```python
from build123d import *

# Parameters (mm, degrees)
SKETCH_1_R               = 2.5
EXTRUDE_1_DEPTH          = 4
SKETCH_3_R               = 7.5
EXTRUDE_3_DEPTH          = 6
SKETCH_4_R               = 10
EXTRUDE_4_DEPTH          = 5
SKETCH_5_R               = 3.175
EXTRUDE_5_DEPTH          = 11
SKETCH_6_R               = 10
EXTRUDE_6_DEPTH          = 5
SKETCH_7_R               = 7.5
EXTRUDE_7_DEPTH          = 7
SKETCH_8_R               = 2.5
EXTRUDE_8_DEPTH          = 4
CUT_EXTRUDE_1_DEPTH      = 45.317039612
CUT_EXTRUDE_1_DEPTH_BACK = 1
SKETCH_10_R              = 2.5
SKETCH_13_R              = 10
SKETCH_13_R_2            = 2.5
CUT_EXTRUDE_3_DEPTH      = 15


with BuildPart() as part:
    # 草图1 → 凸台-拉伸1 (new body)
    with BuildSketch(Plane(origin=(0, 0, 0), x_dir=(1, 0, 0), z_dir=(0, 1, 0))):
        with Locations(Location((0, 0, 0), (0, 0, 270))):
            Circle(SKETCH_1_R)
    extrude(amount=EXTRUDE_1_DEPTH)

    # 草图3 → 凸台-拉伸3 (add)
    with BuildSketch(Plane(origin=(0, 4, 0), x_dir=(1, 0, 0), z_dir=(0, 1, 0))):
        with Locations(Location((0, 0, 0), (0, 0, 270))):
            Circle(SKETCH_3_R)
    extrude(amount=EXTRUDE_3_DEPTH)

    # 草图4 → 凸台-拉伸4 (add)
    with BuildSketch(Plane(origin=(0, 10, 0), x_dir=(1, 0, 0), z_dir=(0, 1, 0))):
        with Locations(Location((0, 0, 0), (0, 0, 270))):
            Circle(SKETCH_4_R)
    extrude(amount=EXTRUDE_4_DEPTH)

    # 草图5 → 凸台-拉伸5 (add)
    with BuildSketch(Plane(origin=(0, 15, 0), x_dir=(1, 0, 0), z_dir=(0, 1, 0))):
        with Locations(Location((0, 0, 0), (0, 0, 270))):
            Circle(SKETCH_5_R)
    extrude(amount=EXTRUDE_5_DEPTH)

    # 草图6 → 凸台-拉伸6 (add)
    with BuildSketch(Plane(origin=(0, 26, 0), x_dir=(1, 0, 0), z_dir=(0, 1, 0))):
        with Locations(Location((0, 0, 0), (0, 0, 270))):
            Circle(SKETCH_6_R)
    extrude(amount=EXTRUDE_6_DEPTH)

    # 草图7 → 凸台-拉伸7 (add)
    with BuildSketch(Plane(origin=(0, 31, 0), x_dir=(1, 0, 0), z_dir=(0, 1, 0))):
        with Locations(Location((0, 0, 0), (0, 0, 270))):
            Circle(SKETCH_7_R)
    extrude(amount=EXTRUDE_7_DEPTH)

    # 草图8 → 凸台-拉伸8 (add)
    with BuildSketch(Plane(origin=(0, 38, 0), x_dir=(1, 0, 0), z_dir=(0, 1, 0))):
        with Locations(Location((0, 0, 0), (0, 0, 270))):
            Circle(SKETCH_8_R)
    extrude(amount=EXTRUDE_8_DEPTH)

    # 草图10 → 切除-拉伸1 (cut, two sides: drawn at the far end of the back side and taken through both)
    with BuildSketch(Plane(origin=(0, 0, 0), x_dir=(-1, 0, 0), z_dir=(0, -1, 0)).offset(-CUT_EXTRUDE_1_DEPTH_BACK)):
        with Locations(Location((0, 0, 0), (0, 0, 90))):
            Circle(SKETCH_10_R)
    extrude(amount=CUT_EXTRUDE_1_DEPTH + CUT_EXTRUDE_1_DEPTH_BACK, mode=Mode.SUBTRACT)

    # 草图13 → 切除-拉伸3 (cut)
    with BuildSketch(Plane.XZ.offset(-26)):
        with Locations(Location((0, 0, 0), (0, 0, 90))):
            Circle(SKETCH_13_R)
        with Locations(Location((0, 0, 0), (0, 0, 270))):
            Circle(SKETCH_13_R_2, mode=Mode.SUBTRACT)
    extrude(amount=-CUT_EXTRUDE_3_DEPTH, mode=Mode.SUBTRACT)


solid = part.part
```
Input: part model. Units: mm. Frame: model coordinates. A direction names the side the tool comes from. Round coordinates to 2 decimals unless told otherwise and drop trailing zeros. Loops run counter-clockwise (first coordinate to the right, second up) from the corner with the lowest first, then second, coordinate; pieces in that order, holes last.
1) Pull-direction query (X, two-part tool) for faces 4 (the cylindrical face through (-1.93, 20.42, -2.52)), 5 (the flat face through (3, 26, 0)); classes: released by +X, released by -X, zero draft, split by the parting line, or undercut.
Ans:
face 4: split by the parting line
face 5: zero draft
2) Section query A-A on z = 0. Return the cut outline in (x, y) (3 decimals).
Ans:
outline: (-10, 10) - (-7.5, 10) - (-7.5, 4) - (-2.5, 4) - (-2.5, 1) - (2.5, 1) - (2.5, 4) - (7.5, 4) - (7.5, 10) - (10, 10) - (10, 15) - (3.175, 15) - (3.175, 26) - (2.5, 26) - (2.5, 42) - (-2.5, 42) - (-2.5, 26) - (-3.175, 26) - (-3.175, 15) - (-10, 15) - close
3) Section query C-C on y = 5. Return the cut outline in (x, z), plus the area to 3 significant figures.
Ans:
outline: circle Ø15 at (0, 0)
area: 177 mm2
4) Set-up query: faces 1 (the cylindrical face through (-2.44, 2.48, -0.54)), 2 (the flat face through (2.4, 15, -2.4)), 3 (the cylindrical face through (-9.76, 12.46, -2.17)). Return all of +Z, -Z, +X, -X, +Y, -Y with unobstructed straight access to the full face (end or side cutting, diameter ignored); none if empty.
Ans:
face 1: -Y
face 2: +Y
face 3: +Y, -Y
5) Pin query (flat end, axial travel): pin 1 (3 mm diameter, centred on y = 6.5, z = -3.5, fed in from -X); pin 2 (4 mm diameter, centred on x = 5.5, y = 6, fed in from +Z); pin 3 (5 mm diameter, centred on x = -4.5, y = 12, fed in from -Z). Return the tip coordinate at first contact, or that it passes through.
Ans:
pin 1: stops at x = -7.23
pin 2: stops at z = 6.63
pin 3: stops at z = -9.8
6) Section query D-D on z = 5.5. Return the cut outline in (x, y).
Ans:
outline: (-8.35, 10) - (-5.1, 10) - (-5.1, 4) - (5.1, 4) - (5.1, 10) - (8.35, 10) - (8.35, 15) - (-8.35, 15) - close
7) Section query B-B on x = -0.75. Return the cut outline in (y, z).
Ans:
outline: (1, -2.38) - (4, -2.38) - (4, -7.46) - (10, -7.46) - (10, -9.97) - (15, -9.97) - (15, -3.09) - (26, -3.09) - (26, -2.38) - (42, -2.38) - (42, 2.38) - (26, 2.38) - (26, 3.09) - (15, 3.09) - (15, 9.97) - (10, 9.97) - (10, 7.46) - (4, 7.46) - (4, 2.38) - (1, 2.38) - close
8) Material intervals for line 1 (Y direction, x = 3.25, z = 8.25); line 2 (Y direction, x = -4.5, z = -0.5); line 3 (Z direction, x = -2.5, y = 21.5), sorted ascending.
Ans:
line 1: y = 10 to 15
line 2: y = 4 to 15
line 3: z = -1.96 to 1.96
